Print and shaded views of the part. All mm, measured from the part's lowest x, y and z. A direction names the side the tool comes from. Give positions to 0.01 mm unless a question says otherwise; leave off trailing zeros. Write each loop counter-clockwise with the first axis right and the second up, starting at its lowest first coordinate (ties: lowest second). Pieces come first, ordered by that corner, then holes. Notation, with made-up numbers: (16, 12) - (71, 12) arc R12 cw to (71, 31) - close; hole circle Ø1 at (55.25, 81.25). An arc over 180 degrees is marked (long way). Use one line per item in the form item = value. Start each with the question number.
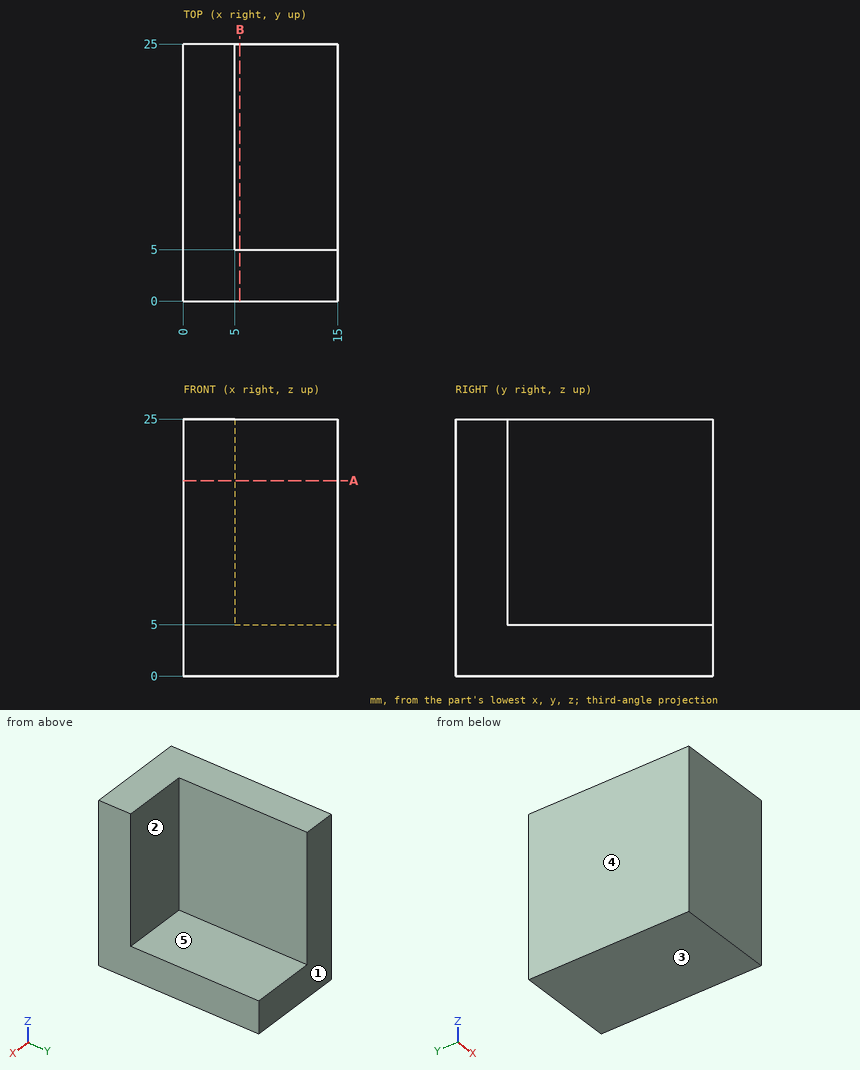
(1) Pin check, flat tips, straight feed: pin 1 Ø6 at (y, z) = (17, 11.5) entering from +X; pin 2 Ø3 at (x, z) = (9, 18) entering from +Y. Stop position of each tip, or through.
(2) Which spindle directions (+Z, -Z, +X, -X, +Y, -Y) get a long thin tool onto all of the face, cutting with end or side? Do the marked faces 1 and 2. Say none if no direction does.
(3) Cut at A-A, the plane z = 19. Give the cut face in (x, y).
(4) Cut at B-B, the plane x = 5.5. Give the cut face in (y, z).
(5) Wall check: line 1 (Y direction, x = 6.75, z = 19.25). Give the ranges that are in metal, low to high. Write a range as from..to.
(6) Two-plate mould, pull along Z, no slides. Class the marked faces 3, 4 and 5: +Z half, -Z half, draft (parallel to the pull), parting line (faces both ways), or undercut.
Solution:
q1.pin_1 = 5
q1.pin_2 = 5
q2.face_1 = +Z, -Z, +X, -X, +Y
q2.face_2 = +Z, +X, +Y
q3.outline = (0, 0) - (15, 0) - (15, 5) - (5, 5) - (5, 25) - (0, 25) - close
q4.outline = (0, 0) - (25, 0) - (25, 5) - (5, 5) - (5, 25) - (0, 25) - close
q5.line_1 = 0..5
q6.face_3 = -Z half
q6.face_4 = draft
q6.face_5 = +Z half
